from build123d import *

# Parameters (mm, degrees)
BOSS_EXTRUDE1_DEPTH      = 34
BOSS_EXTRUDE1_DEPTH_BACK = 34
SKETCH2_R                = 12.5
KEYWAY_DEPTH             = 71.525832556
CHAMFER1_SIZE            = 0.79375


with BuildPart() as part:
    # Sketch2 → Boss-Extrude1 (new, two sides: drawn at the far end of the back side and taken through both)
    with BuildSketch(Plane.XY.offset(-BOSS_EXTRUDE1_DEPTH_BACK)):
        Circle(SKETCH2_R)
    extrude(amount=BOSS_EXTRUDE1_DEPTH + BOSS_EXTRUDE1_DEPTH_BACK)

    # KeySketch → Keyway (cut, through all)
    with BuildSketch(Plane(origin=(-0.021590267, -1.396144607, 34), x_dir=(1, 0, 0), z_dir=(0, 0, 1))):
        with BuildLine():
            Line((-2.359659733, 8.968037019), (-2.359659733, 11.467244607))
            Line((-2.359659733, 11.467244607), (2.402840267, 11.467244607))
            Line((2.402840267, 11.467244607), (2.402840267, 8.968037019))
            ThreePointArc((2.402840267, 8.968037019), (0.021590267, -6.541355393), (-2.359659733, 8.968037019))
        make_face()
    extrude(amount=-KEYWAY_DEPTH, mode=Mode.SUBTRACT)

    # Chamfer1
    chamfer1_edges = [part.edges().sort_by_distance(p)[0] for p in [
        (0, -7.9375, -34),
        (0, -7.9375, 34),
    ]]
    chamfer(chamfer1_edges, length=CHAMFER1_SIZE)


solid = part.part
Work out the finished part from the listing and answer in its coordinate system (mm). A direction names the side the tool comes from. Give positions to 0.01 mm unless a question says otherwise; leave off trailing zeros. Write each loop counter-clockwise with the first axis right and the second up, starting at its lowest first coordinate (ties: lowest second). Pieces come first, ordered by that corner, then holes. Notation, with made-up numbers: (37.25, -14) - (68.25, -14) arc R20 cw to (68.25, 8) - close; hole circle Ø10 at (20.25, 88.5). An arc over 180 degrees is marked (long way). One line per item, written item: value. Start each with the question number.
1. Consider probe 1 along Y at (x, z) = (0, -11); probe 2 along Y at (x, z) = (-5, -24.5); probe 3 along X at (y, z) = (-6.5, -27.5). Determine where each line is inside the solid, lowest interval first.
2. Find section A-A (y = 0). Write down the section's boundary in (x, z).
3. Find section C-C (z = -13). Write down the section's boundary in (x, y) (1 decimal).
4. For a pull along X with two mould halves and no side action, classify faces 3 (the flat face through (-9, -3, 34)), 4 (the conical face through (-0.323, -8.058, -33.333)), 5 (the cylindrical face through (11.923, 3.755, -0.476)) as +X half, -X half, draft (parallel to the pull), parting line (faces both ways), or undercut.
5. Find section D-D (x = 10.75). Write down the section's boundary in (y, z), then the cut area to 4 significant figures.
6. For faces 1 (the flat face through (2.381, 9, 0)), 2 (the flat face through (-9, -3, -34)), determine the directions among +Z, -Z, +X, -X, +Y, -Y from which every point of the face is accessible in a straight line to the end or side of a thin tool.
7. Given pin 1 (2 mm diameter, centred on x = -7.5, z = 17, fed in from +Y); pin 2 (0.7 mm diameter, centred on y = 9, z = 2, fed in from +X); pin 3 (1.5 mm diameter, centred on y = -6.5, z = 10, fed in from -X), each flat-ended and moving along its own axis, determine where each tip first touches the part or whether it passes through.
8. Find section B-B (x = 0). Write down the section's boundary in (y, z).
Geometry results:
1. probe 1: -12.5 to -7.94, 10.07 to 12.5
1. probe 2: -11.46 to -6.16, 6.16 to 11.46
1. probe 3: -10.68 to -4.56, 4.56 to 10.68
2. outline: (-12.5, -34) - (-8.73, -34) - (-7.94, -33.21) - (-7.94, 33.21) - (-8.73, 34) - (-12.5, 34) - close; (7.94, -33.21) - (8.73, -34) - (12.5, -34) - (12.5, 34) - (8.73, 34) - (7.94, 33.21) - close
3. outline: circle Ø25 at (0, 0); hole (-2.4, 7.6) arc R7.9 ccw (long way) to (2.4, 7.6) - (2.4, 10.1) - (-2.4, 10.1) - close
4. face 3: draft
4. face 4: undercut
4. face 5: parting line
5. outline: (-6.38, -34) - (6.38, -34) - (6.38, 34) - (-6.38, 34) - close
5. area: 867.5 mm2
6. face 1: +Z, -Z
6. face 2: -Z, +X, -X, +Y, -Y
7. pin 1: y = 10.68
7. pin 2: x = 9.02
7. pin 3: x = -11.1
8. outline: (-12.5, -34) - (-8.73, -34) - (-7.94, -33.21) - (-7.94, 33.21) - (-8.73, 34) - (-12.5, 34) - close; (10.07, -34) - (12.5, -34) - (12.5, 34) - (10.07, 34) - close
